```python
from build123d import *

# Parameters (mm, degrees)
BOSS_EXTRUDE1_DEPTH     = 5
SKETCH2_R               = 1
CUT_EXTRUDE1_DEPTH      = 15
SHELL1_DEPTH            = 3.5
SKETCH4_R               = 2.25
CUT_EXTRUDE2_DEPTH      = 3
FILLET2_R               = 3
BOSS_EXTRUDE2_DEPTH     = 5
CUT_EXTRUDE3_DEPTH      = 3.5
SKETCH8_W               = 3.515564437
SKETCH8_H               = 15
BOSS_EXTRUDE3_DEPTH     = 3
SKETCH9_R               = 2
CUT_EXTRUDE5_DEPTH      = 3
FILLET3_R               = 10
CUT_EXTRUDE7_DEPTH      = 3
CUT_EXTRUDE7_DEPTH_BACK = 1.5
BOSS_EXTRUDE4_START     = 3.5
BOSS_EXTRUDE4_DEPTH     = 3.5


with BuildPart() as part:
    # Sketch1 → Boss-Extrude1 (new body)
    with BuildSketch(Plane(origin=(0, 0, 0), x_dir=(1, 0, 0), z_dir=(0, 1, 0))):
        with BuildLine():
            Line((-8, 10), (8, 10))
            ThreePointArc((8, 10), (9.414213562, 9.414213562), (10, 8))
            Line((10, 8), (10, -8))
            ThreePointArc((10, -8), (9.414213562, -9.414213562), (8, -10))
            Line((8, -10), (-8, -10))
            ThreePointArc((-8, -10), (-9.414213562, -9.414213562), (-10, -8))
            Line((-10, -8), (-10, 8))
            ThreePointArc((-10, 8), (-9.414213562, 9.414213562), (-8, 10))
        make_face()
    extrude(amount=BOSS_EXTRUDE1_DEPTH)

    # Sketch2 → Cut-Extrude1 (cut)
    with BuildSketch(Plane.XZ):
        with Locations(Location((-8.5, 8.5, 0), (0, 0, 270))):
            Circle(SKETCH2_R)
        with Locations(Location((8.5, 8.5, 0), (0, 0, 270))):
            Circle(SKETCH2_R)
        with Locations(Location((8.5, -8.5, 0), (0, 0, 270))):
            Circle(SKETCH2_R)
        with Locations(Location((-8.5, -8.5, 0), (0, 0, 270))):
            Circle(SKETCH2_R)
    extrude(amount=-CUT_EXTRUDE1_DEPTH, mode=Mode.SUBTRACT)

    # Shell1: read off the stored shape, not the designer's step
    # Shell1 outline → Shell1 (cut)
    with BuildSketch(Plane(origin=(0, 0, 0), x_dir=(1, 0, 0), z_dir=(0, 1, 0))):
        with BuildLine():
            Line((6, 8.5), (-6, 8.5))
            ThreePointArc((-6, 8.5), (-6.732233047, 6.732233047), (-8.5, 6))
            Line((-8.5, 6), (-8.5, -6))
            ThreePointArc((-8.5, -6), (-6.732233047, -6.732233047), (-6, -8.5))
            Line((-6, -8.5), (6, -8.5))
            ThreePointArc((6, -8.5), (6.732233047, -6.732233047), (8.5, -6))
            Line((8.5, -6), (8.5, 6))
            ThreePointArc((8.5, 6), (6.732233047, 6.732233047), (6, 8.5))
        make_face()
    extrude(amount=SHELL1_DEPTH, mode=Mode.SUBTRACT)

    # Sketch4 → Cut-Extrude2 (cut)
    with BuildSketch(Plane(origin=(0, 5, 0), x_dir=(1, 0, 0), z_dir=(0, 1, 0))):
        with Locations((8.5, -8.5)):
            Circle(SKETCH4_R)
        with Locations((-8.5, -8.5)):
            Circle(SKETCH4_R)
        with Locations((-8.5, 8.5)):
            Circle(SKETCH4_R)
        with Locations((8.5, 8.5)):
            Circle(SKETCH4_R)
    extrude(amount=-CUT_EXTRUDE2_DEPTH, mode=Mode.SUBTRACT)

    # Fillet2
    fillet2_edges = [part.edges().sort_by_distance(p)[0] for p in [
        (6.822949017, 3.5, -10),
        (10, 3.5, -6.822949017),
        (-6.822949017, 3.5, -10),
        (-10, 3.5, -6.822949017),
        (-10, 3.5, 6.822949017),
        (-6.822949017, 3.5, 10),
        (6.822949017, 3.5, 10),
        (10, 3.5, 6.822949017),
    ]]
    fillet(fillet2_edges, radius=FILLET2_R)

    # Sketch5 → Boss-Extrude2 (add)
    with BuildSketch(Plane.XZ):
        with BuildLine():
            Line((10, 7.5), (14, 7.5))
            ThreePointArc((14, 7.5), (15.414213562, 6.914213562), (16, 5.5))
            Line((16, 5.5), (16, -5.5))
            ThreePointArc((16, -5.5), (15.414213562, -6.914213562), (14, -7.5))
            Line((14, -7.5), (10, -7.5))
            Line((10, -7.5), (10, 7.5))
        make_face()
    extrude(amount=-BOSS_EXTRUDE2_DEPTH)

    # Sketch6 → Cut-Extrude3 (cut)
    with BuildSketch(Plane.XZ):
        with BuildLine():
            Line((8.5, 5.5), (13, 5.5))
            ThreePointArc((13, 5.5), (14.060660172, 5.060660172), (14.5, 4))
            Line((14.5, 4), (14.5, -4))
            ThreePointArc((14.5, -4), (14.060660172, -5.060660172), (13, -5.5))
            Line((13, -5.5), (8.5, -5.5))
            Line((8.5, -5.5), (8.5, 5.5))
        make_face()
    extrude(amount=-CUT_EXTRUDE3_DEPTH, mode=Mode.SUBTRACT)

    # Sketch8 → Boss-Extrude3 (add)
    with BuildSketch(Plane(origin=(0, 5, 0), x_dir=(1, 0, 0), z_dir=(0, 1, 0))):
        with Locations((8.242217782, 0)):
            Rectangle(SKETCH8_W, SKETCH8_H)
    extrude(amount=-BOSS_EXTRUDE3_DEPTH)

    # Sketch9 → Cut-Extrude5 (cut)
    with BuildSketch(Plane(origin=(0, 5, 0), x_dir=(1, 0, 0), z_dir=(0, 1, 0))):
        with Locations((8.5, 8.5)):
            Circle(SKETCH9_R)
        with Locations((8.5, -8.5)):
            Circle(SKETCH9_R)
    extrude(amount=-CUT_EXTRUDE5_DEPTH, mode=Mode.SUBTRACT)

    # Fillet3
    # the kernel refuses this fillet: 10 mm, written as the material it takes off along each edge
    with BuildSketch(Plane(origin=(10.232050808, 2, -7.5), x_dir=(1, 0, 0), z_dir=(0, 1, 0))) as fillet3_piece_1:
        with BuildLine():
            CenterArc((3.063780716, -10), FILLET3_R, 90, 23.556464309)
            ThreePointArc((-0.932745554, -0.833333333), (-0.399552407, -0.491458351), (0, 0))
            Line((0, 0), (3.063780716, 0))
        make_face()
    extrude(amount=10.659451789, mode=Mode.SUBTRACT)
    with BuildSketch(Plane(origin=(6.767949192, 2, -7.5), x_dir=(0.649978972407837, 0, 0.759952192856664), z_dir=(0, 1, 0))) as fillet3_piece_2:
        with BuildLine():
            CenterArc((2.560910878, -9.831273909), FILLET3_R, 100.540016502, 5.393327967)
            Line((-0.184277898, -0.215456804), (0, 0))
            ThreePointArc((0, 0), (0.365844411, -0.033745218), (0.731688822, 0))
        make_face()
    extrude(amount=4.829222056, mode=Mode.SUBTRACT)
    with BuildSketch(Plane(origin=(10.232050808, 2, 7.5), x_dir=(-0.7457291752746819, 0, -0.6662492004829293), z_dir=(0, 1, 0))) as fillet3_piece_3:
        with BuildLine():
            CenterArc((4.377741338, -9.498533205), FILLET3_R, 108.221767845, 23.556464309)
            Line((-2.284750666, -2.041241452), (0, 0))
            ThreePointArc((0, 0), (0.62539162, -0.100293359), (1.25078324, 0))
        make_face()
    extrude(amount=10.659451789, mode=Mode.SUBTRACT)
    with BuildSketch(Plane(origin=(6.767949192, 2, 7.5), x_dir=(-1.0, 0, -2.3874717233974133e-11), z_dir=(0, 1, 0))) as fillet3_piece_4:
        with BuildLine():
            CenterArc((5.806759945, -8.33629115), FILLET3_R, 123.52663903, 5.393327967)
            ThreePointArc((-0.475582349, -0.556048525), (-0.212146422, -0.299957945), (0, 0))
            Line((0, 0), (0.28351363, 0))
        make_face()
    extrude(amount=4.829222056, mode=Mode.SUBTRACT)

    # Sketch10 → Cut-Extrude7 (cut, two sides: drawn at the far end of the back side and taken through both)
    with BuildSketch(Plane.XZ.offset(-2).offset(-CUT_EXTRUDE7_DEPTH_BACK)):
        with BuildLine():
            Line((8.5, 6), (13, 6))
            ThreePointArc((13, 6), (14.060660172, 5.560660172), (14.5, 4.5))
            Line((14.5, 4.5), (14.5, -4.5))
            ThreePointArc((14.5, -4.5), (14.060660172, -5.560660172), (13, -6))
            Line((13, -6), (8.5, -6))
            ThreePointArc((8.5, -6), (7.370298682, -6.269803835), (6.484435563, -7.020980054))
            Line((6.484435563, -7.020980054), (6.484435563, 7.020980054))
            ThreePointArc((6.484435563, 7.020980054), (7.392428114, 6.313490581), (8.5, 6))
        make_face()
    extrude(amount=CUT_EXTRUDE7_DEPTH + CUT_EXTRUDE7_DEPTH_BACK, mode=Mode.SUBTRACT)

    # Sketch11 → Boss-Extrude4 (add)
    with BuildSketch(Plane.XZ.offset(-3.5).offset(BOSS_EXTRUDE4_START)):
        with BuildLine():
            Line((4.951661673, -8.5), (6, -8.5))
            ThreePointArc((6, -8.5), (6.732233047, -6.732233047), (8.5, -6))
            Line((8.5, -6), (11.018075631, -6))
            ThreePointArc((11.018075631, -6), (7.148016159, -5.219322543), (4.951661673, -8.5))
        make_face()
        with BuildLine():
            Line((11.018075631, 6), (8.5, 6))
            ThreePointArc((8.5, 6), (6.798059889, 6.798059889), (6, 8.5))
            Line((6, 8.5), (4.951661673, 8.5))
            ThreePointArc((4.951661673, 8.5), (7.148016159, 5.219322543), (11.018075631, 6))
        make_face()
        with BuildLine():
            Line((-6, 8.5), (-5.487129131, 8.5))
            ThreePointArc((-5.487129131, 8.5), (-6.369578578, 6.369578578), (-8.5, 5.487129131))
            Line((-8.5, 5.487129131), (-8.5, 6))
            ThreePointArc((-8.5, 6), (-6.732233047, 6.732233047), (-6, 8.5))
        make_face()
        with BuildLine():
            Line((-8.5, -6), (-8.5, -5.487129131))
            ThreePointArc((-8.5, -5.487129131), (-6.365781058, -6.365781058), (-5.487129131, -8.5))
            Line((-5.487129131, -8.5), (-5.689784623, -8.747525568))
            Line((-5.689784623, -8.747525568), (-6, -8.5))
            ThreePointArc((-6, -8.5), (-6.728431484, -6.728431484), (-8.5, -6))
        make_face()
    extrude(amount=-BOSS_EXTRUDE4_DEPTH)


solid = part.part
```
Build history of the part. All positions in model axes, mm. A direction names the side the tool comes from. Round coordinates to 2 decimals unless told otherwise and drop trailing zeros. Write each loop counter-clockwise with the first axis right and the second up, starting at its lowest first coordinate (ties: lowest second). Pieces come first, ordered by that corner, then holes. Notation, with made-up numbers: (13, 81) - (45, 81) arc R21 cw to (45, 112) - close; hole circle Ø9 at (-33.5, 50). An arc over 180 degrees is marked (long way). Answer as CSV lines item,"result".
Q1. Cut at C-C (x = 8.5). Write the cut outline in (y, z).
Report:
outline,"(0, -9.94) - (2, -9.94) - (2, -9.5) - (0, -9.5) - close; (0, -7.5) - (2, -7.5) - (2, -6.5) - (5, -6.5) - (5, 6.5) - (2, 6.5) - (2, 7.5) - (0, 7.5) - (0, 4.95) - (3.5, 4.95) - (3.5, -4.95) - (0, -4.95) - close; (0, 9.5) - (2, 9.5) - (2, 9.94) - (0, 9.94) - close"
Q2. Tool access for faces 1 (the flat face through (12, 1, 7.5)), 2 (the cylindrical face through (14.05, 1.77, 5.57)), 3 (the flat face through (12, 1, -7.5)), 4 (the cylindrical face through (-6.9, 3.52, 6.92)), 5 (the cylindrical face through (8.22, 3.52, -6.52)): list every direction of +Z, -Z, +X, -X, +Y, -Y with a clear straight run to the whole face (end or side of a thin tool).
Report:
face 1,"+Z, +X, +Y, -Y"
face 2,"-Y"
face 3,"-Z, +X, +Y, -Y"
face 4,"+Z, -X, +Y"
face 5,"-Z, +Y"
Q3. Drop flat-ended pins along their axis: pin 1 (8.5 mm diameter, centred on x = 4.5, z = -3, fed in from -Y); pin 2 (1.2 mm diameter, centred on x = 8.5, z = 8.5, fed in from -Y); pin 3 (0.6 mm diameter, centred on y = 1, z = -7.5, fed in from +X); pin 4 (1 mm diameter, centred on x = 12, y = 1, fed in from -Z). Give the stop position or say it passes through.
Report:
pin 1,"stops at y = 0"
pin 2,"passes through"
pin 3,"stops at x = 15.05"
pin 4,"stops at z = -7.5"
Q4. Cut at D-D (x = -2.25). Write the cut outline in (y, z), and give its area (3 significant figures).
Report:
outline,"(0, -10) - (5, -10) - (5, 10) - (0, 10) - (0, 8.5) - (3.5, 8.5) - (3.5, -8.5) - (0, -8.5) - close"
area,"40.5 mm^2"
Q5. Cut at A-A (y = 0.7). State how many separate pieces and enclosed holes the cut face has, and give its area (3 significant figures).
Report:
separate pieces,"1"
enclosed holes,"6"
area,"150 mm^2"
Q6. Pull direction X, two halves, no side cores. Call faces 6 (the cylindrical face through (7.2, 1.7, -5.2)), 7 (the cylindrical face through (15.4, 2.46, 6.93)), 8 (the flat face through (7, 0, -7)): +X half, -X half, draft (parallel to the pull), parting line (faces both ways), or undercut.
Report:
face 6,"undercut"
face 7,"+X half"
face 8,"draft"
Q7. Drill centre lines: probe 1 along Z at (x, y) = (1, 0.3); probe 2 along X at (y, z) = (2.75, 3.25); probe 3 along Z at (x, y) = (11.5, 0.8). Where is each one in solid material? Low to high. Write a range as [from, to].
Report:
probe 1,"z = [-10, -8.5], [8.5, 10]"
probe 2,"x = [-10, -8.5], [14.5, 16]"
probe 3,"z = [-7.5, -6], [6, 7.5]"
Q8. Cut at B-B (z = -0.25). Write the cut outline in (x, y).
Report:
outline,"(-10, 0) - (-8.5, 0) - (-8.5, 3.5) - (14.5, 3.5) - (14.5, 0) - (16, 0) - (16, 5) - (-10, 5) - close"
